from build123d import *

# Parameters (mm, degrees)
F1_DEPTH = 25.4
F2_R     = 50.8
F3_DEPTH = 25.4
F4_W     = 63.5
F4_H     = 38.1
F5_DEPTH = 25.4


with BuildPart() as f1:
    # F0 (on Top) → F1 (new body)
    with BuildSketch(Plane.XY):
        with BuildLine():
            Line((-75.701751, 0), (76.2, 0))
            ThreePointArc((76.2, 0), (0, 76.2), (-76.2, 0))
            Line((-76.2, 0), (-75.701751, 0))
        make_face()
        with BuildLine():
            ThreePointArc((-75.701751, -8.699708), (4.356982, -76.075336), (76.2, 0))
            Line((76.2, 0), (-75.701751, 0))
            Line((-75.701751, 0), (-75.701751, -8.699708))
        make_face()
        with BuildLine():
            Line((76.2, -101.6), (76.2, 0))
            ThreePointArc((76.2, 0), (4.356982, -76.075336), (-75.701751, -8.699708))
            Line((-75.701751, -8.699708), (-75.701751, -101.6))
            Line((-75.701751, -101.6), (76.2, -101.6))
        make_face()
    extrude(amount=F1_DEPTH)

    # F2 (on face) → F3 (cut)
    with BuildSketch(Plane.XY.offset(25.4)):
        Circle(F2_R)
    extrude(amount=-F3_DEPTH, mode=Mode.SUBTRACT)

    # F4 (on face) → F5 (cut)
    with BuildSketch(Plane.XY.offset(25.4)):
        with Locations((0, -82.55)):
            Rectangle(F4_W, F4_H)
    extrude(amount=-F5_DEPTH, mode=Mode.SUBTRACT)


solid = f1.part
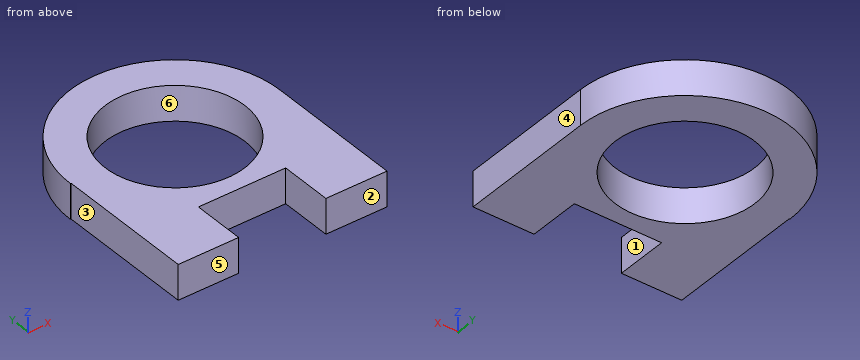
Here's how the part is built. I have some questions about the finished solid (model axes, mm). Face numbers are marked on the shaded views. A direction names the side the tool comes from. Give positions to 0.01 mm unless a question says otherwise; leave off trailing zeros. Loops run counter-clockwise (first coordinate to the right, second up) from the corner with the lowest first, then second, coordinate; pieces in that order, holes last. Notation, with made-up numbers: (-19, 5.25) -> (5, 5.25) arc R30 ccw to (5, 40.25) -> close; hole circle Ø9 at (-32.5, -5). An arc over 180 degrees is marked (long way). Answer as a JSON object with one key per item and string values. Group by question number.
Item 1: Imagine slicing it at B-B on z = 12.25. Write out the boundary of the cut face in (x, y), then the cut area to 3 significant figures.
Item 2: I need wall thicknesses on L1, parallel to Y at x = 0, z = 15.75; L2, parallel to X at y = -81, z = 24.25; L3, parallel to X at y = -8.5, z = 24. Which ranges of each line are inside material? Lowest first, please.
Item 3: Imagine slicing it at C-C on y = 43. Write out the boundary of the cut face in (x, z), then the cut area to 3 significant figures.
Item 4: Imagine slicing it at D-D on x = 56. Write out the boundary of the cut face in (y, z), then the cut area to 3 significant figures.
Item 5: Will these pins go through, and if not, where does the flat tip stop? pin 1 (12 mm diameter, centred on x = -9, z = 9.5, fed in from -Y); pin 2 (3 mm diameter, centred on y = 16, z = 18.5, fed in from -X); pin 3 (3 mm diameter, centred on y = 5.5, z = 13, fed in from +X).
Item 6: Imagine slicing it at A-A on x = 0. Write out the boundary of the cut face in (y, z).
Item 7: Thinking about a two-plate mould opening in X: for the marked faces 4, 5 and 6, which applies, pulls with the +X half, pulls with the -X half, needs draft (parallel to the pull), parting line crosses it, or undercut?
Item 8: On a 3-axis mill with a long thin cutter (end or side, diameter ignored), from which of +Z, -Z, +X, -X, +Y, -Y can I reach the whole of each face in a straight line? I mean the marked faces 1, 2 and 3. Say none if no direction works.
Answer list:
{
 "1": {"outline": "(-76.2, 0) -> (-75.7, 0) -> (-75.7, -101.6) -> (-31.75, -101.6) -> (-31.75, -63.5) -> (31.75, -63.5) -> (31.75, -101.6) -> (76.2, -101.6) -> (76.2, 0) arc R76.2 ccw to start; hole circle Ø101.6 at (0, 0)", "area": "14,000 mm2"},
 "2": {"L1": "y = -63.5 to -50.8, 50.8 to 76.2", "L2": "x = -75.7 to -31.75, 31.75 to 76.2", "L3": "x = -75.7 to -50.08, 50.08 to 76.2"},
 "3": {"outline": "(-62.91, 0) -> (-27.05, 0) -> (-27.05, 25.4) -> (-62.91, 25.4) -> close; (27.05, 0) -> (62.91, 0) -> (62.91, 25.4) -> (27.05, 25.4) -> close", "area": "1,820 mm2"},
 "4": {"outline": "(-101.6, 0) -> (51.68, 0) -> (51.68, 25.4) -> (-101.6, 25.4) -> close", "area": "3,890 mm2"},
 "5": {"pin 1": "stops at y = -63.5", "pin 2": "stops at x = -74.81", "pin 3": "stops at x = 76.09"},
 "6": {"outline": "(-63.5, 0) -> (-50.8, 0) -> (-50.8, 25.4) -> (-63.5, 25.4) -> close; (50.8, 0) -> (76.2, 0) -> (76.2, 25.4) -> (50.8, 25.4) -> close"},
 "7": {"face 4": "pulls with the +X half", "face 5": "needs draft", "face 6": "undercut"},
 "8": {"face 1": "+Z, -Z, -Y", "face 2": "+Z, -Z, +X, -X, -Y", "face 3": "+Z, -Z, -X, -Y"}
}
